Read the model definition and answer for the solid it produces. Units are mm, in the model's axes. A direction names the side the tool comes from. Coordinates: 2 decimals unless noted, no trailing zeros. Write each loop counter-clockwise with the first axis right and the second up, starting at its lowest first coordinate (ties: lowest second). Pieces come first, ordered by that corner, then holes.
Item 1: Section A-A (z = 1.5) is taken. State how many separate pieces and enclosed holes the cut face has, then the cut area to 3 significant figures.
Item 2: Each of these flat-tipped pins is pushed along its axis until it touches: P1, Ø2, axis at x = 4.135, y = -13.45, coming from the +Z side (3 decimals); P2, Ø0.7, axis at x = -10, y = 1.5, coming from the +Z side (3 decimals); P3, Ø6, axis at y = 2.5, z = 1, coming from the +X side. Where does it stop, or does it pass through?
Item 3: Section D-D (z = -5.75) is taken. Give the vertices of the cut face in (x, y).
Item 4: A tool of negligible diameter and unlimited length cuts with its end or side. For faces 1 (the face through (10.2, 1.7, -2.865)), 2 (the face through (10.23, 4.17, -0.04)), 3 (the face through (-0.98, -12, -3)), 4 (the face through (3.143, -14.211, -4.321)), from which of +Z, -Z, +X, -X, +Y, -Y can it reach the whole face along a straight path? Write none if from no direction.
Item 5: Determine the mould class of faces 5 (the face through (0, 7, -7.6)), 6 (the face through (6.485, -11.8, 4.3)), 7 (the face through (4, -8.2, 3)) for opening direction Z: released by +Z, released by -Z, zero draft, split by the parting line, or undercut.
Item 6: Section C-C (x = 1) is taken. Give the vertices of the cut face in (y, z) (3 decimals).
Item 7: Straight lines are drawn through the part: probe 1 along X at (y, z) = (-13.45, -4.05) (3 decimals); probe 2 along Z at (x, y) = (-7, -11) (3 decimals); probe 3 along X at (y, z) = (0.25, -2). For each, find the intervals that lie inside material, in ascending order.
from build123d import *

# Parameters (mm, degrees)
SKETCH_1_W          = 18.5
SKETCH_1_H          = 16.4
EXTRUDE_1_DEPTH     = 6.35
SKETCH_2_W          = 21.7
SKETCH_2_H          = 15.2
EXTRUDE_2_DEPTH     = 2.3
EXTRUDE_3_DEPTH     = 2.865
EXTRUDE_4_DEPTH     = 7.3
SKETCH_5_W          = 4.7
SKETCH_5_H          = 0.81
SKETCH_5_H_2        = 0.82
EXTRUDE_5_DEPTH     = 8.25
CHAMFER_1_SIZE      = 1
SKETCH_6_R          = 1.25
CUT_EXTRUDE_1_DEPTH = 2.25
EXTRUDE_6_DEPTH     = 4.125
SKETCH_8_W          = 15.4
SKETCH_8_H          = 8.65
SKETCH_8_W_2        = 15
SKETCH_8_H_2        = 8.25
CUT_EXTRUDE_2_DEPTH = 1


with BuildPart() as part:
    # 草图1 → 凸台-拉伸1 (new body, symmetric)
    with BuildSketch(Plane.XY):
        Rectangle(SKETCH_1_W, SKETCH_1_H)
    extrude(amount=EXTRUDE_1_DEPTH, both=True)

    # 草图2 → 凸台-拉伸2 (add)
    with BuildSketch(Plane(origin=(0, 8.2, 0), x_dir=(1, 0, 0), z_dir=(0, 1, 0))):
        Rectangle(SKETCH_2_W, SKETCH_2_H)
    extrude(amount=-EXTRUDE_2_DEPTH)

    # 草图3 → 凸台-拉伸3 (add, symmetric)
    with BuildSketch(Plane.XY):
        Polygon((9.25, 5.9), (9.767443892, 5.9), (10.7, 2.4), (9.25, -4.1), (9.25, -1.80352853), (10.185361465, 2.389471142), align=None)
        Polygon((-10.185361465, 2.389471142), (-9.25, 5.9), (-9.767443892, 5.9), (-10.7, 2.4), (-9.25, -4.1), (-9.25, -1.80352853), align=None)
    extrude(amount=EXTRUDE_3_DEPTH, both=True)

    # 草图4 → 凸台-拉伸4 (add)
    with BuildSketch(Plane.XZ.offset(8.2)):
        Polygon((-9.25, 0.525), (-2.03, 0.525), (-2.03, 6.35), (-0.98, 6.35), (-0.98, 0.525), (9.25, 0.525), (9.25, -0.525), (-0.98, -0.525), (-0.98, -6.35), (-2.03, -6.35), (-2.03, -0.525), (-9.25, -0.525), align=None)
    extrude(amount=EXTRUDE_4_DEPTH)

    # 草图5 → 凸台-拉伸5 (add)
    with BuildSketch(Plane.XZ.offset(8.2)):
        with Locations((-5.64, 3.12)):
            Rectangle(SKETCH_5_W, SKETCH_5_H)
        with Locations((4.135, 4.315)):
            Rectangle(SKETCH_5_W, SKETCH_5_H_2)
        with Locations((4.135, -4.315)):
            Rectangle(SKETCH_5_W, SKETCH_5_H_2)
        with Locations((-5.64, -3.12)):
            Rectangle(SKETCH_5_W, SKETCH_5_H)
    extrude(amount=EXTRUDE_5_DEPTH)

    # 倒角1
    chamfer_1_edges = [part.edges().sort_by_distance(p)[0] for p in [
        (-3.29, -16.45, 3.12),
        (-7.99, -16.45, 3.12),
        (6.485, -16.45, 4.315),
        (1.785, -16.45, 4.315),
        (1.785, -16.45, -4.315),
        (6.485, -16.45, -4.315),
        (-7.99, -16.45, -3.12),
        (-3.29, -16.45, -3.12),
    ]]
    chamfer(chamfer_1_edges, length=CHAMFER_1_SIZE)

    # 草图6 → 切除-拉伸1 (cut)
    with BuildSketch(Plane.XY.offset(4.725)):
        with Locations((4.135, -13.45)):
            Circle(SKETCH_6_R)
        with Locations((-5.64, -13.45)):
            Circle(SKETCH_6_R)
    cut_extrude_1 = extrude(amount=-CUT_EXTRUDE_1_DEPTH, mode=Mode.SUBTRACT)

    # 镜向1: 切除-拉伸1 across plane
    add(cut_extrude_1.mirror(Plane.XY), mode=Mode.SUBTRACT)

    # 草图7 → 凸台-拉伸6 (add, symmetric)
    with BuildSketch(Plane.XY):
        with BuildLine():
            ThreePointArc((5, 13.2), (6.484981539, 10.817490769), (7.5, 8.2))
            Line((7.5, 8.2), (-7.5, 8.2))
            ThreePointArc((-7.5, 8.2), (-0.764940017, 9.487350042), (5, 13.2))
        make_face()
    extrude(amount=EXTRUDE_6_DEPTH, both=True)

    # 草图8 → 切除-拉伸2 (cut)
    with BuildSketch(Plane(origin=(0, 8.2, 0), x_dir=(1, 0, 0), z_dir=(0, 1, 0))):
        Rectangle(SKETCH_8_W, SKETCH_8_H)
        Rectangle(SKETCH_8_W_2, SKETCH_8_H_2, mode=Mode.SUBTRACT)
    extrude(amount=-CUT_EXTRUDE_2_DEPTH, mode=Mode.SUBTRACT)


solid = part.part
Established:
1. separate pieces: 1
1. enclosed holes: 2
1. area: 354 mm2
2. P1: stops at z = 0.525
2. P2: stops at z = 2.865
2. P3: stops at x = 10.7
3. outline: (-10.85, 5.9) - (-9.25, 5.9) - (-9.25, -8.2) - (-2.03, -8.2) - (-2.03, -15.5) - (-0.98, -15.5) - (-0.98, -8.2) - (9.25, -8.2) - (9.25, 5.9) - (10.85, 5.9) - (10.85, 8.2) - (-10.85, 8.2) - close
4. face 1: -Z, +X, -Y
4. face 2: +Z, -Z, +X
4. face 3: -Z, -Y
4. face 4: -Z
5. face 5: released by -Z
5. face 6: zero draft
5. face 7: undercut
6. outline: (-15.5, -0.525) - (-8.2, -0.525) - (-8.2, -6.35) - (5.9, -6.35) - (5.9, -7.6) - (8.2, -7.6) - (8.2, -4.325) - (7.2, -4.325) - (7.2, -4.125) - (10.307, -4.125) - (10.307, 4.125) - (7.2, 4.125) - (7.2, 4.325) - (8.2, 4.325) - (8.2, 7.6) - (5.9, 7.6) - (5.9, 6.35) - (-8.2, 6.35) - (-8.2, 0.525) - (-15.5, 0.525) - close
7. probe 1: x = -2.03 to -0.98, 1.785 to 2.885, 5.385 to 6.485
7. probe 2: z = -3.525 to -2.715, -0.525 to 0.525, 2.715 to 3.525
7. probe 3: x = -10.22 to -9.71, -9.25 to 9.25, 9.71 to 10.22
